Could you check a few things on this model? Use its own coordinates, in mm. A direction names the side the tool comes from. Give positions to 0.01 mm unless a question says otherwise; leave off trailing zeros. Write each loop counter-clockwise with the first axis right and the second up, starting at its lowest first coordinate (ties: lowest second). Pieces come first, ordered by that corner, then holes. Notation, with made-up numbers: (-29, -26.5) - (3, -26.5) arc R33 ccw to (3, 6.5) - close; hole circle Ø9 at (7.5, 43.25). An arc over 180 degrees is marked (long way). Answer as CSV lines item,"result". Start each with the question number.
Q1. Imagine slicing it at B-B on x = 3.75. List the corners of the cut face in (y, z) for me.
Q2. We'd pull the mould along X, two halves only. Please class faces 1 (the face through (-8.128, 0, 2)), 2 (the face through (0, 1, 0.864)), 3 (the face through (-0.1, -2.4, 0)): pulls with the +X half, pulls with the -X half, needs draft (parallel to the pull), parting line crosses it, or undercut.
Q3. Imagine slicing it at C-C on y = -1.25. List the corners of the cut face in (x, z) for me.
Q4. Will these pins go through, and if not, where does the flat tip stop? pin 1 Ø2 at (y, z) = (0.5, -2.5) entering from +X; pin 2 Ø2.5 at (x, z) = (-0.5, -4) entering from -Y; pin 3 Ø0.8 at (y, z) = (-0.5, 2.5) entering from -X.
Q5. Imagine slicing it at A-A on z = -3.25. List the corners of the cut face in (x, y) for me, and give its area (3 significant figures).
Q6. On a 3-axis mill with a long thin cutter (end or side, diameter ignored), from which of +Z, -Z, +X, -X, +Y, -Y can I reach the whole of each face in a straight line? I mean faces 4 (the face through (7.544, -2.4, -2.4)), 5 (the face through (6.782, -2.4, -2.7)), 6 (the face through (0, -0.8, 2)), 7 (the face through (8.128, 0, 2)). Say none if no direction works.
Q7. Imagine slicing it at D-D on x = -7.75. List the corners of the cut face in (y, z) for me.
Q8. If I drill on line 1 along X through (y, z) = (-2.45, -4.75); line 2 along Z through (x, y) = (-1.25, 2.25); line 3 along Y through (x, z) = (-3.25, -0.75), over which ranges is the centre line in solid material (lowest first)?
Autodesk Inventor part; units mm, degrees
ref_plane "YZ Plane" through (0, 0, 0) normal (1, 0, 0) x (0, 1, 0)
ref_plane "XZ Plane" through (0, 0, 0) normal (0, 1, 0) x (-1, 0, 0)
ref_plane "XY Plane" through (0, 0, 0) normal (0, 0, 1) x (1, 0, 0)
sketch "Sketch1" plane through (0, 0, 0) normal (0, 0, 1) x (1, 0, 0)
  line L0 (-9.144, 1.9939) -> (9.144, 1.9939)
  line L1 (9.144, 1.9939) -> (9.144, -1.9939)
  line L2 (9.144, -1.9939) -> (-9.144, -1.9939)
  line L3 (-9.144, -1.9939) -> (-9.144, 1.9939)
  line L4 (-9.144, 1.9939) -> (9.144, -1.9939) construction
  line L5 (9.144, 1.9939) -> (-9.144, -1.9939) construction
  line L6 (-9.8806, 2.7305) -> (9.8806, 2.7305)
  line L7 (9.8806, 2.7305) -> (9.8806, -1.9939)
  line L8 (9.8806, -1.9939) -> (-9.8806, -1.9939)
  line L9 (-9.8806, -1.9939) -> (-9.8806, 2.7305)
  line L10 (-7.5438, -1.9939) -> (-6.7818, -1.9939)
  line L11 (-6.7818, -1.9939) -> (-6.7818, -2.8829)
  line L12 (-6.7818, -2.8829) -> (-7.5438, -2.8829)
  line L13 (-7.5438, -2.8829) -> (-7.5438, -1.9939)
  line L14 (-7.5438, -2.8829) -> (7.5438, -2.8829)
  line L15 (7.5438, -2.8829) -> (7.5438, -1.9939)
  line L16 (7.5438, -1.9939) -> (-7.5438, -1.9939)
  line L17 (-7.5438, -1.9939) -> (-7.5438, -2.8829)
  line L18 (7.5438, -1.9939) -> (6.7818, -1.9939)
  line L19 (6.7818, -1.9939) -> (6.7818, -2.8829)
  line L20 (6.7818, -2.8829) -> (7.5438, -2.8829)
  line L21 (7.5438, -2.8829) -> (7.5438, -1.9939)
  line L22 (0, 0) -> (0, -2.8829) construction
  dimension "d0" = 18.288
  dimension "d1" = 3.9878
  dimension "d4" = 0.7366
  dimension "d6" = 0.7366
  dimension "d7" = 0.7366
  dimension "d14" = 0.762
  dimension "d16" = 0.889
  dimension "d17" = 13.5636
extrude "Extrusion1" add sketch "Sketch1" against normal blind 7.2136 contours L0 L1 L2 L3
extrude "Extrusion2" add sketch "Sketch1" along normal blind 0.8636
sketch "Sketch2" plane through (0, 0, 0.8636) normal (0, 0, 1) x (1, 0, 0)
  line L0 (-8.128, 0.8001) -> (8.128, 0.8001)
  line L1 (8.128, 0.8001) -> (8.128, -0.8001)
  line L2 (8.128, -0.8001) -> (-8.128, -0.8001)
  line L3 (-8.128, -0.8001) -> (-8.128, 0.8001)
  line L4 (8.128, 0.8001) -> (-8.128, -0.8001) construction
  point P0 (0, 0)
  point P1 (0, 0)
  dimension "d10" = 16.256
  dimension "d11" = 1.6002
extrude "Extrusion3" add sketch "Sketch2" along normal blind 2.54
extrude "Extrusion4" add sketch "Sketch1" against normal blind 5.5372 contours L2 L11 L12 L13 | L15 L14 L19 L2
properties part number "jst-xh 7c"
Conclusion:
1,outline,"(-2.88, 0) - (-1.99, 0) - (-1.99, -7.21) - (1.99, -7.21) - (1.99, 0) - (2.73, 0) - (2.73, 0.86) - (0.8, 0.86) - (0.8, 3.4) - (-0.8, 3.4) - (-0.8, 0.86) - (-2.88, 0.86) - close"
2,face 1,"pulls with the -X half"
2,face 2,"needs draft"
2,face 3,"undercut"
3,outline,"(-9.88, 0) - (-9.14, 0) - (-9.14, -7.21) - (9.14, -7.21) - (9.14, 0) - (9.88, 0) - (9.88, 0.86) - (-9.88, 0.86) - close"
4,pin 1,"x = 9.14"
4,pin 2,"y = -1.99"
4,pin 3,"x = -8.13"
5,outline,"(-9.14, -1.99) - (-7.54, -1.99) - (-7.54, -2.88) - (-6.78, -2.88) - (-6.78, -1.99) - (6.78, -1.99) - (6.78, -2.88) - (7.54, -2.88) - (7.54, -1.99) - (9.14, -1.99) - (9.14, 1.99) - (-9.14, 1.99) - close"
5,area,"74.3 mm^2"
6,face 4,"+Z, -Z, +X, -Y"
6,face 5,"-Z, -Y"
6,face 6,"+Z, +X, -X, -Y"
6,face 7,"+Z, +X, +Y, -Y"
7,outline,"(-1.99, -7.21) - (1.99, -7.21) - (1.99, 0) - (2.73, 0) - (2.73, 0.86) - (0.8, 0.86) - (0.8, 3.4) - (-0.8, 3.4) - (-0.8, 0.86) - (-1.99, 0.86) - close"
8,line 1,"-7.54 to -6.78, 6.78 to 7.54"
8,line 2,"0 to 0.86"
8,line 3,"-1.99 to 1.99"
